The listing builds one solid part. Answer for the finished solid, in the listing's coordinates (mm). A direction names the side the tool comes from. Give positions to 0.01 mm unless a question says otherwise; leave off trailing zeros. Write each loop counter-clockwise with the first axis right and the second up, starting at its lowest first coordinate (ties: lowest second). Pieces come first, ordered by that corner, then holes. Notation, with made-up numbers: (31, 88.25) -> (52, 88.25) arc R13 cw to (52, 102.25) -> close; hole circle Ø3 at (13, 32). An arc over 180 degrees is marked (long way). Put each result on its own line as item: value. Start each with the question number.
1) Find the intervals of material crossed by line 1 along Y through (x, z) = (0, 9.8); line 2 along Y through (x, z) = (0, 8.25), in increasing order. Write a range as from..to.
2) For faces 4 (the cylindrical face through (25.73, 13.38, 9.75)), 5 (the cylindrical face through (-7.1, 22.4, 0.2)), 6 (the flat face through (-26.1, -13.1, 0)), determine the directions among +Z, -Z, +X, -X, +Y, -Y from which every point of the face is accessible in a straight line to the end or side of a thin tool.
3) A cutting plane is placed at C-C (z = 6.75). Write down the section's boundary in (x, y).
4) For a pull along Y with two mould halves and no side action, classify faces 1 (the cylindrical face through (21, -28, 5)), 2 (the flat face through (-24, 0, 9.5)), 3 (the flat face through (-26.1, -13.1, 10)) as released by +Y, released by -Y, zero draft, split by the parting line, or undercut.
5) A cutting plane is placed at A-A (y = 0). Write down the section's boundary in (x, z), then the cut area to 3 significant figures.
6) Flat-ended cylindrical pins translate along their axes: pin 1 Ø2 at (y, z) = (-24.5, 3) entering from -X; pin 2 Ø6 at (y, z) = (-3, 7.5) entering from +X; pin 3 Ø2 at (y, z) = (24.5, 5.5) entering from +X. Find the tip coordinate at first contact, or state that the pin passes through.
7) A cutting plane is placed at D-D (y = -20.5). Write down the section's boundary in (x, z).
from build123d import *

# Parameters (mm, degrees)
SKETCH1_R             = 23.5
SKETCH1_R_2           = 17.5
BOSS_EXTRUDE1_DEPTH   = 10
SKETCH1_R_3           = 35
SKETCH1_R_4           = 29
BOSS_EXTRUDE1_2_DEPTH = 10
BOSS_EXTRUDE2_START   = 0.5
SKETCH1_3_R           = 29
SKETCH1_3_R_2         = 23.5
BOSS_EXTRUDE2_DEPTH   = 9


with BuildPart() as part:
    # Sketch1 → Boss-Extrude1 (new body)
    with BuildSketch(Plane(origin=(0, 0, 0), x_dir=(0, 1, 0), z_dir=(0, 0, 1))):
        Circle(SKETCH1_R)
        Circle(SKETCH1_R_2, mode=Mode.SUBTRACT)
    extrude(amount=BOSS_EXTRUDE1_DEPTH)



with BuildPart() as body_2:
    # Sketch1 → Boss-Extrude1 2 (new body)
    with BuildSketch(Plane(origin=(0, 0, 0), x_dir=(0, 1, 0), z_dir=(0, 0, 1))):
        Circle(SKETCH1_R_3)
        Circle(SKETCH1_R_4, mode=Mode.SUBTRACT)
    extrude(amount=BOSS_EXTRUDE1_2_DEPTH)


with BuildPart() as part_1:
    add(part.part)

    add(body_2.part)  # Boss-Extrude2 merges body 2
    # Sketch1_3 → Boss-Extrude2 (add)
    with BuildSketch(Plane(origin=(0, 0, 0), x_dir=(0, 1, 0), z_dir=(0, 0, 1)).offset(BOSS_EXTRUDE2_START)):
        Circle(SKETCH1_3_R)
        Circle(SKETCH1_3_R_2, mode=Mode.SUBTRACT)
    extrude(amount=BOSS_EXTRUDE2_DEPTH)


solid = part_1.part
Reply:
1. line 1: y = -35..-29, -23.5..-17.5, 17.5..23.5, 29..35
1. line 2: y = -35..-17.5, 17.5..35
2. face 4: +Z
2. face 5: -Z
2. face 6: -Z, +X, -X, +Y, -Y
3. outline: circle Ø70 at (0, 0); hole circle Ø35 at (0, 0)
4. face 1: split by the parting line
4. face 2: undercut
4. face 3: zero draft
5. outline: (-35, 0) -> (-29, 0) -> (-29, 0.5) -> (-23.5, 0.5) -> (-23.5, 0) -> (-17.5, 0) -> (-17.5, 10) -> (-23.5, 10) -> (-23.5, 9.5) -> (-29, 9.5) -> (-29, 10) -> (-35, 10) -> close; (17.5, 0) -> (23.5, 0) -> (23.5, 0.5) -> (29, 0.5) -> (29, 0) -> (35, 0) -> (35, 10) -> (29, 10) -> (29, 9.5) -> (23.5, 9.5) -> (23.5, 10) -> (17.5, 10) -> close
5. area: 339 mm2
6. pin 1: stops at x = -25.94
6. pin 2: stops at x = 35
6. pin 3: stops at x = 25.94
7. outline: (-28.37, 0) -> (-20.51, 0) -> (-20.51, 0.5) -> (-11.49, 0.5) -> (-11.49, 0) -> (11.49, 0) -> (11.49, 0.5) -> (20.51, 0.5) -> (20.51, 0) -> (28.37, 0) -> (28.37, 10) -> (20.51, 10) -> (20.51, 9.5) -> (11.49, 9.5) -> (11.49, 10) -> (-11.49, 10) -> (-11.49, 9.5) -> (-20.51, 9.5) -> (-20.51, 10) -> (-28.37, 10) -> close
